Here's the drawing with two shaded views (mm, measured from the low corner). I have some questions. Give positions to 0.01 mm unless a question says otherwise; leave off trailing zeros. Loops run counter-clockwise (first coordinate to the right, second up) from the corner with the lowest first, then second, coordinate; pieces in that order, holes last. Notation, with made-up numbers: M 16,35.25 L 61,35.25 A21 ccw 61,58.25 Z; hole C 66.25,87.5 d7. An arc over 180 degrees is marked long. Use a Markdown table: item, result. Add a question column.
1) Suppose I cut it at A-A on z = 5. List the corners of the cut face in (x, y) for me (3 decimals), and give its area (3 significant figures).
2) Suppose I cut it at B-B on z = 45. List the corners of the cut face in (x, y) for me (3 decimals), and give its area (3 significant figures).
3) Will these pins go through, and if not, where does the flat tip stop? pin 1 Ø4 at (y, z) = (14.125, 5) entering from +X; pin 2 Ø3 at (x, z) = (7, 13) entering from -Y.
4) If I drill on line 1 along Y through (x, z) = (8.25, 5) (3 decimals); line 2 along Z through (x, y) = (8, 13.5); line 3 along Y through (x, z) = (16.75, 6.5) (3 decimals), over which ranges is the centre line in solid material (lowest first)? Write a range as [from, to].
5) Suppose I cut it at D-D on y = 18.75. List the corners of the cut face in (x, z) for me, and give its area (3 significant figures).
6) Suppose I cut it at C-C on x = 14.5. List the corners of the cut face in (y, z) for me (3 decimals).
7) We'd pull the mould along Y, two halves only. Please class the marked faces 1, 2 and 3: +Y half, -Y half, draft (parallel to the pull), parting line (faces both ways), or undercut.
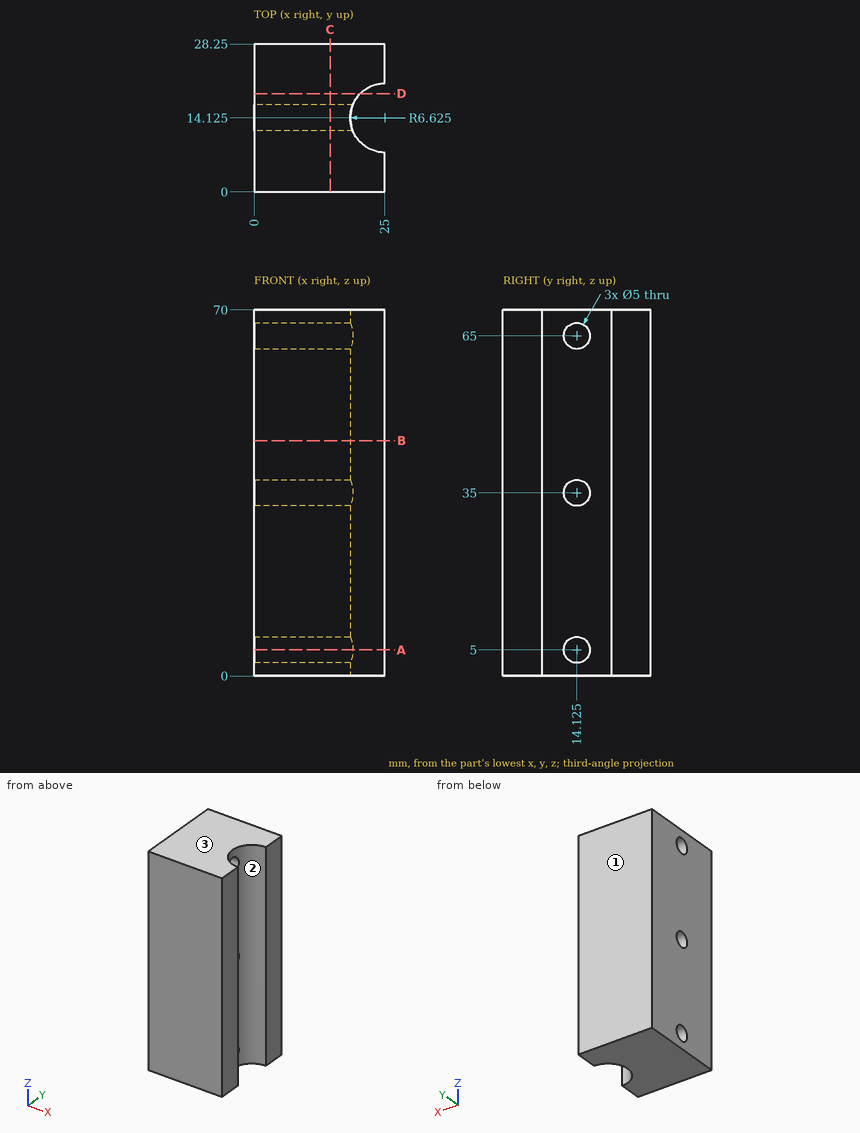
Answer block:
| question | item | result |
|---|---|---|
| 1 | outline | M 0,0 L 25,0 L 25,7.5 A6.625 cw 18.865,11.625 L 0,11.625 Z; M 0,16.625 L 18.865,16.625 A6.625 cw 25,20.75 L 25,28.25 L 0,28.25 Z |
| 1 | area | 545 mm^2 |
| 2 | outline | M 0,0 L 25,0 L 25,7.5 A6.625 cw 25,20.75 L 25,28.25 L 0,28.25 Z |
| 2 | area | 637 mm^2 |
| 3 | pin 1 | passes through |
| 3 | pin 2 | stops at y = 0 |
| 4 | line 1 | y = [0, 11.625], [16.625, 28.25] |
| 4 | line 2 | z = [0, 2.58], [7.42, 32.58], [37.42, 62.58], [67.42, 70] |
| 4 | line 3 | y = [0, 12.125], [16.125, 28.25] |
| 5 | outline | M 0,0 L 20.26,0 L 20.26,70 L 0,70 Z |
| 5 | area | 1,420 mm^2 |
| 6 | outline | M 0,0 L 28.25,0 L 28.25,70 L 0,70 Z; hole C 14.125,5 d5; hole C 14.125,35 d5; hole C 14.125,65 d5 |
| 7 | face 1 | +Y half |
| 7 | face 2 | undercut |
| 7 | face 3 | draft |
